```python
from build123d import *

# Parameters (mm, degrees)
SKETCH1_R           = 8
BOSS_EXTRUDE1_DEPTH = 16
SKETCH2_W           = 88
SKETCH2_H           = 57
BOSS_EXTRUDE2_DEPTH = 10
SKETCH3_R           = 8
BOSS_EXTRUDE3_DEPTH = 16
SKETCH4_R           = 27.5
BOSS_EXTRUDE4_DEPTH = 38
CUT_EXTRUDE2_DEPTH  = 92.105707834


with BuildPart() as part:
    # Sketch1 → Boss-Extrude1 (new body)
    with BuildSketch(Plane.XY):
        with BuildLine():
            Line((-28, 28.5), (-28, -28.5))
            Line((-28, -28.5), (-18, -28.5))
            Line((-18, -28.5), (7.793097747, -12.816693314))
            ThreePointArc((7.793097747, -12.816693314), (15, 0), (7.793097747, 12.816693314))
            Line((7.793097747, 12.816693314), (-18, 28.5))
            Line((-18, 28.5), (-28, 28.5))
        make_face()
        Circle(SKETCH1_R, mode=Mode.SUBTRACT)
    extrude(amount=-BOSS_EXTRUDE1_DEPTH)

    # Sketch2 → Boss-Extrude2 (add)
    with BuildSketch(Plane.ZY.offset(28)):
        with Locations((28, 0)):
            Rectangle(SKETCH2_W, SKETCH2_H)
    extrude(amount=-BOSS_EXTRUDE2_DEPTH)

    # Sketch3 → Boss-Extrude3 (add)
    with BuildSketch(Plane.XY.offset(72)):
        with BuildLine():
            Line((7.793097747, 12.816693314), (-18, 28.5))
            Line((-18, 28.5), (-18, -28.5))
            Line((-18, -28.5), (7.793097747, -12.816693314))
            ThreePointArc((7.793097747, -12.816693314), (15, 0), (7.793097747, 12.816693314))
        make_face()
        Circle(SKETCH3_R, mode=Mode.SUBTRACT)
    extrude(amount=-BOSS_EXTRUDE3_DEPTH)

    # Sketch4 → Boss-Extrude4 (add)
    with BuildSketch(Plane.ZY.offset(28)):
        with Locations((28, 0)):
            Circle(SKETCH4_R)
        with BuildLine():
            Line((47, 4), (47, -4))
            Line((47, -4), (42.456832295, -4))
            ThreePointArc((42.456832295, -4), (13, 0), (42.456832295, 4))
            Line((42.456832295, 4), (47, 4))
        make_face(mode=Mode.SUBTRACT)
    extrude(amount=BOSS_EXTRUDE4_DEPTH)

    # Sketch5 → Cut-Extrude2 (cut, through all)
    with BuildSketch(Plane(origin=(-18, 0, 0), x_dir=(0, 0, -1), z_dir=(1, 0, 0))):
        with BuildLine():
            Line((-47, -4), (-47, 4))
            Line((-47, 4), (-42.456832295, 4))
            ThreePointArc((-42.456832295, 4), (-13, 0), (-42.456832295, -4))
            Line((-42.456832295, -4), (-47, -4))
        make_face()
    extrude(amount=-CUT_EXTRUDE2_DEPTH, mode=Mode.SUBTRACT)


solid = part.part
```
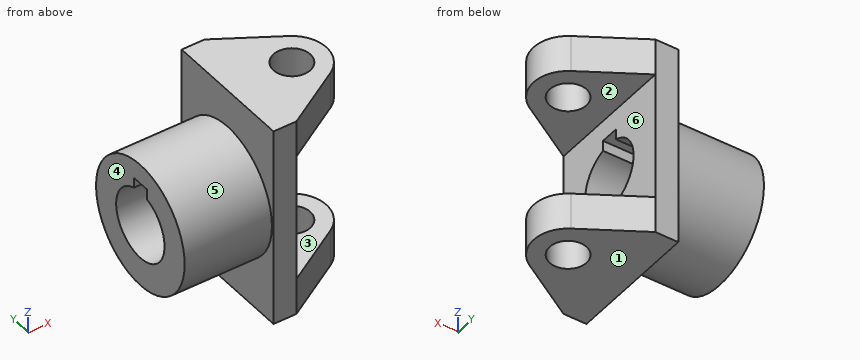
Model file for the job. Use its own axes, mm. Face numbers are marked on the shaded views. A direction names the side the tool comes from. Coordinates: 2 decimals unless noted, no trailing zeros. Loops run counter-clockwise (first coordinate to the right, second up) from the corner with the lowest first, then second, coordinate; pieces in that order, holes last. Notation, with made-up numbers: (13.5, 24.5) -> (25.5, 24.5) arc R16 cw to (25.5, 37.5) -> close; hole circle Ø7 at (-32.75, -26.5). An arc over 180 degrees is marked (long way). Answer as a JSON object with one key per item and string values.
Q1. Cut at C-C (x = -46.5). List the corners of the cut face in (y, z).
Report:
{"outline": "circle Ø55 at (0, 28); hole (-4, 42.46) arc R15 ccw (long way) to (4, 42.46) -> (4, 47) -> (-4, 47) -> close"}
Q2. Cut at D-D (x = 0). List the corners of the cut face in (y, z), and give its area (3 significant figures).
Report:
{"outline": "(-17.56, -16) -> (-8, -16) -> (-8, 0) -> (-17.56, 0) -> close; (-17.56, 56) -> (-8, 56) -> (-8, 72) -> (-17.56, 72) -> close; (8, -16) -> (17.56, -16) -> (17.56, 0) -> (8, 0) -> close; (8, 56) -> (17.56, 56) -> (17.56, 72) -> (8, 72) -> close", "area": "612 mm2"}
Q3. Flat gauge pins, fed straight in: P1, Ø2, axis at y = 18, z = 8, coming from the +X side; P2, Ø4, axis at x = -41.5, z = 0.5, coming from the -Y side; P3, Ø2, axis at y = 6.5, z = -0.5, coming from the -X side. Where does each tip first touch, or does it go through?
Report:
{"P1": "stops at x = -18", "P2": "stops at y = -10.3", "P3": "stops at x = -28"}
Q4. 3-axis set-ups, long thin cutter, end or side, ignore diameter. For the marked faces 1 and 2: which of +Z, -Z, +X, -X, +Y, -Y reach the whole face in a straight line?
Report:
{"face 1": "-Z, +X, -X, +Y, -Y", "face 2": "+X, +Y, -Y"}
Q5. Cut at B-B (z = 28). List the corners of the cut face in (x, y), and give its area (3 significant figures).
Report:
{"outline": "(-66, -27.5) -> (-28, -27.5) -> (-28, -28.5) -> (-18, -28.5) -> (-18, -15) -> (-66, -15) -> close; (-66, 15) -> (-18, 15) -> (-18, 28.5) -> (-28, 28.5) -> (-28, 27.5) -> (-66, 27.5) -> close", "area": "1,220 mm2"}
Q6. Cut at A-A (y = 0). List the corners of the cut face in (x, z).
Report:
{"outline": "(-66, 0.5) -> (-28, 0.5) -> (-28, -16) -> (-8, -16) -> (-8, 0) -> (-18, 0) -> (-18, 13) -> (-66, 13) -> close; (-66, 47) -> (-18, 47) -> (-18, 56) -> (-8, 56) -> (-8, 72) -> (-28, 72) -> (-28, 55.5) -> (-66, 55.5) -> close; (8, -16) -> (15, -16) -> (15, 0) -> (8, 0) -> close; (8, 56) -> (15, 56) -> (15, 72) -> (8, 72) -> close"}
Q7. Probe probe 1 along Z at (x, y) = (3.5, -13); probe 2 along Y at (x, z) = (-29, 28); probe 3 along Z at (x, y) = (-47.5, -5). List the from-to ranges inside material, lowest first.
Report:
{"probe 1": "z = -16 to 0, 56 to 72", "probe 2": "y = -27.5 to -15, 15 to 27.5", "probe 3": "z = 0.96 to 13.86, 42.14 to 55.04"}
Q8. Pull direction Z, two halves, no side cores. Call the marked faces 3, 4, 5 and 6: released by +Z, released by -Z, zero draft, split by the parting line, or undercut.
Report:
{"face 3": "undercut", "face 4": "zero draft", "face 5": "split by the parting line", "face 6": "undercut"}
